from build123d import *

# Parameters (mm, degrees)
F0_W     = 1
F0_H     = 163.5
F1_DEPTH = 6
F0_W_2   = 0.7
F2_R     = 0.5
F2_2_R   = 0.5
F0_W_3   = 3.9
F3_DEPTH = 1


with BuildPart() as f1:
    # F0 (on Top) → F1 (new body)
    with BuildSketch(Plane.XY):
        with Locations((-2.45, 61.75)):
            Rectangle(F0_W, F0_H)
    extrude(amount=F1_DEPTH)

    # F2
    f2_edges = [f1.edges().sort_by_distance(p)[0] for p in [
        (-2.95, 61.75, 6),
        (-2.95, 61.75, 0),
    ]]
    fillet(f2_edges, radius=F2_R)



with BuildPart() as f1b:
    # F0 (on Top) → F1, piece 2 (new body)
    with BuildSketch(Plane.XY):
        with Locations((2.3, 61.75)):
            Rectangle(F0_W_2, F0_H)
    extrude(amount=F1_DEPTH)

    # F2#2
    f2_2_edges = [f1b.edges().sort_by_distance(p)[0] for p in [
        (2.65, 61.75, 6),
        (2.65, 61.75, 0),
    ]]
    fillet(f2_2_edges, radius=F2_2_R)


with BuildPart() as f1_1:
    add(f1.part)

    add(f1b.part)  # F3 merges F1b
    # F0 (on Top) → F3 (join)
    with BuildSketch(Plane.XY):
        with Locations((0, 61.75)):
            Rectangle(F0_W_3, F0_H)
    extrude(amount=F3_DEPTH)


solid = f1_1.part
Model file for the job. Use its own axes, mm. A direction names the side the tool comes from. Give positions to 0.01 mm unless a question says otherwise; leave off trailing zeros. Loops run counter-clockwise (first coordinate to the right, second up) from the corner with the lowest first, then second, coordinate; pieces in that order, holes last. Notation, with made-up numbers: (-35.5, 16.25) -> (-7.5, 16.25) arc R16 ccw to (-7.5, 44.25) -> close; hole circle Ø1 at (46, -36.75). An arc over 180 degrees is marked (long way). Use a Markdown table: item, result. Add a question column.
(1) Tool access for faces 1 (the flat face through (2.65, 61, 3)), 2 (the flat face through (1.95, 61, 3)): list every direction of +Z, -Z, +X, -X, +Y, -Y with a clear straight run to the whole face (end or side of a thin tool).
(2) Slice it at A-A on z = 2.25. List the corners of the cut face in (x, y).
(3) Drop a flat-ended pin along its axis: pin 1 Ø1 at (x, z) = (-1, 2) entering from -Y. Give the stop position or say it passes through.
(4) Slice it at C-C on x = 0.65. List the corners of the cut face in (y, z), and give its area (4 significant figures).
(5) Slice it at B-B on y = 95. List the corners of the cut face in (x, z), and give its area (3 significant figures).
(6) Wall check: line 1 along X through (y, z) = (109.5, 2.85); line 2 along Z through (x, y) = (0.15, 90). Give the ranges that are in metal, low to high.
Filled sheet:
| question | item | result |
|---|---|---|
| 1 | face 1 | +Z, -Z, +X, +Y, -Y |
| 1 | face 2 | +Z, +Y, -Y |
| 2 | outline | (-2.95, -20) -> (-1.95, -20) -> (-1.95, 143.5) -> (-2.95, 143.5) -> close; (1.95, -20) -> (2.65, -20) -> (2.65, 143.5) -> (1.95, 143.5) -> close |
| 3 | pin 1 | through |
| 4 | outline | (-20, 0) -> (143.5, 0) -> (143.5, 1) -> (-20, 1) -> close |
| 4 | area | 163.5 mm2 |
| 5 | outline | (-2.95, 0.5) arc R0.5 ccw to (-2.45, 0) -> (2.15, 0) arc R0.5 ccw to (2.65, 0.5) -> (2.65, 5.5) arc R0.5 ccw to (2.15, 6) -> (1.95, 6) -> (1.95, 1) -> (-1.95, 1) -> (-1.95, 6) -> (-2.45, 6) arc R0.5 ccw to (-2.95, 5.5) -> close |
| 5 | area | 13.9 mm2 |
| 6 | line 1 | -2.95 to -1.95, 1.95 to 2.65 |
| 6 | line 2 | 0 to 1 |
